from build123d import *

# Parameters (mm, degrees)
F1_DEPTH = 38.1
F3_DEPTH = 25.4
F5_DEPTH = 25.4


with BuildPart() as f1:
    # F0 (on Right) → F1 (new body)
    with BuildSketch(Plane.YZ):
        Polygon((-12.276925, 5.197683), (-12.276925, 43.297683), (-24.976925, 43.297683), (-24.976925, 17.897683), (-37.676925, 17.897683), (-37.676925, 5.197683), align=None)
    extrude(amount=F1_DEPTH)

    # F2 (on face) → F3 (cut)
    with BuildSketch(Plane.XZ.offset(24.976925)):
        Polygon((38.1, 43.297683), (25.4, 43.297683), (38.1, 17.897683), align=None)
    extrude(amount=-F3_DEPTH, mode=Mode.SUBTRACT)

    # F4 (on face) → F5 (cut)
    with BuildSketch(Plane.XY.offset(17.897683)):
        Polygon((38.1, -37.676925), (38.1, -24.976925), (25.4, -37.676925), align=None)
    extrude(amount=-F5_DEPTH, mode=Mode.SUBTRACT)


solid = f1.part
Work out the finished part from the listing and answer in its coordinate system (mm). A direction names the side the tool comes from. Coordinates: 2 decimals unless noted, no trailing zeros. Loops run counter-clockwise (first coordinate to the right, second up) from the corner with the lowest first, then second, coordinate; pieces in that order, holes last. Notation, with made-up numbers: (72, 8) -> (129, 8) arc R36 ccw to (129, 47) -> close; hole circle Ø7 at (-8.5, -19). An arc over 180 degrees is marked (long way). Answer as CSV lines item,"result".
1) The part is cut by section A-A (y = -21.25). Give the vertices of the cut face in (x, z), and give its area (3 significant figures).
A:
outline,"(0, 5.2) -> (38.1, 5.2) -> (38.1, 17.9) -> (25.4, 43.3) -> (0, 43.3) -> close"
area,"1,290 mm²"
2) The part is cut by section D-D (x = 17.5). Give the vertices of the cut face in (y, z).
A:
outline,"(-37.68, 5.2) -> (-12.28, 5.2) -> (-12.28, 43.3) -> (-24.98, 43.3) -> (-24.98, 17.9) -> (-37.68, 17.9) -> close"
3) The part is cut by section B-B (z = 15). Give the vertices of the cut face in (x, y), and give its area (3 significant figures).
A:
outline,"(0, -37.68) -> (25.4, -37.68) -> (38.1, -24.98) -> (38.1, -12.28) -> (0, -12.28) -> close"
area,"887 mm²"
4) For faces 1 (the face through (13, -19, 43.298)), 2 (the face through (15, -31, 17.898)), determine the directions among +Z, -Z, +X, -X, +Y, -Y from which every point of the face is accessible in a straight line to the end or side of a thin tool.
A:
face 1,"+Z, +X, -X, +Y, -Y"
face 2,"+Z, +X, -X, -Y"
5) Straight lines are drawn through the part: probe 1 along Y at (x, z) = (6.5, 21.5); probe 2 along Z at (x, y) = (14, -26); probe 3 along Z at (x, y) = (30.5, -17). For each, find the intervals that lie inside material, in ascending order.
A:
probe 1,"y = -24.98 to -12.28"
probe 2,"z = 5.2 to 17.9"
probe 3,"z = 5.2 to 33.1"
6) Flat-ended cylindrical pins translate along their axes: pin 1 (7.5 mm diameter, centred on x = 10, z = 33, fed in from -Y); pin 2 (6.5 mm diameter, centred on x = 11, y = -32, fed in from +Z). Find the tip coordinate at first contact, or state that the pin passes through.
A:
pin 1,"stops at y = -24.98"
pin 2,"stops at z = 17.9"
7) The part is cut by section C-C (x = 31.5). Give the vertices of the cut face in (y, z), and give its area (3 significant figures).
A:
outline,"(-31.58, 5.2) -> (-12.28, 5.2) -> (-12.28, 31.1) -> (-24.98, 31.1) -> (-24.98, 17.9) -> (-31.58, 17.9) -> close"
area,"413 mm²"
